from build123d import *

# Parameters (mm, degrees)
F0_R            = 76.2
F1_DEPTH        = 76
F2_R            = 44.704
F3_DEPTH        = 50
F4_R            = 6
F5_DEPTH        = 76
F5_COPIES_COUNT = 6


# Not quite as in the source:
# - a pattern or mirror of a feature is missing from the dataset's text; its kind, count and spacing are read off the source's solid


with BuildPart() as f1:
    # F0 (on Top) → F1 (new body)
    with BuildSketch(Plane.XY):
        Circle(F0_R)
    extrude(amount=F1_DEPTH)

    # F2 (on face) → F3 (cut)
    with BuildSketch(Plane(origin=(0, 0, 0), x_dir=(1, 0, 0), z_dir=(0, 0, -1))):
        Circle(F2_R)
    extrude(amount=-F3_DEPTH, mode=Mode.SUBTRACT)

    # F4 (on face) → F5 (cut)
    with BuildSketch(Plane.XY.offset(76)):
        with Locations((-65, 0)):
            Circle(F4_R)
    f5 = extrude(amount=-F5_DEPTH, mode=Mode.SUBTRACT)

    # F5_copies: F5 ×6 about axis
    f5_copies_axis = Axis((0, 0, 0), (0, 0, 1))
    for i in range(1, F5_COPIES_COUNT):
        add(f5.rotate(f5_copies_axis, i * 360 / F5_COPIES_COUNT), mode=Mode.SUBTRACT)


solid = f1.part
Geometry check sheet. Reference: the model listing, model coordinates, mm. A direction names the side the tool comes from. Coordinates: 2 decimals unless noted, no trailing zeros. Write each loop counter-clockwise with the first axis right and the second up, starting at its lowest first coordinate (ties: lowest second). Pieces come first, ordered by that corner, then holes. Notation, with made-up numbers: (-6, 4) -> (25, 4) arc R21 cw to (25, 22) -> close; hole circle Ø7 at (75, 89.5). An arc over 180 degrees is marked (long way). One line per question, with ' | ' between items.
1. Cross-section at D-D on x = -32.5. Record the cut outline in (y, z).
Answers:
outline: (-68.92, 0) -> (-62.29, 0) -> (-62.29, 76) -> (-68.92, 76) -> close; (-50.29, 0) -> (-30.7, 0) -> (-30.7, 50) -> (30.7, 50) -> (30.7, 0) -> (50.29, 0) -> (50.29, 76) -> (-50.29, 76) -> close; (62.29, 0) -> (68.92, 0) -> (68.92, 76) -> (62.29, 76) -> close
2. Depth check by flat-ended pin: pin 1 Ø8 at (x, z) = (32, 53) entering from -Y; pin 2 Ø2 at (y, z) = (34, 18) entering from +X; pin 3 Ø8 at (x, y) = (38.5, 5) entering from -Z. Enter the tip coordinate at first touch or a pass-through.
Answers:
pin 1: stops at y = -70.87 | pin 2: stops at x = 68.68 | pin 3: stops at z = 50
3. Thickness scan on probe 1 along X at (y, z) = (-0.5, 12); probe 2 along Y at (x, z) = (0, 28); probe 3 along X at (y, z) = (3, 27). Record the ranges inside material, lowest first. Write a range as from..to.
Answers:
probe 1: x = -76.2..-70.98, -59.02..-44.7, 44.7..59.02, 70.98..76.2 | probe 2: y = -76.2..-44.7, 44.7..76.2 | probe 3: x = -76.14..-70.2, -59.8..-44.6, 44.6..59.8, 70.2..76.14
4. Set-up check for faces 4 (the cylindrical face through (-35.476, 27.202, 24.65)), 5 (the cylindrical face through (27.74, 52.64, 38.53)): record each of +Z, -Z, +X, -X, +Y, -Y from which the full face is reachable in a straight line by a thin tool's end or side.
Answers:
face 4: -Z | face 5: +Z, -Z
5. Cross-section at C-C on z = 16.5. Record the cut outline in (x, y).
Answers:
outline: circle Ø152.4 at (0, 0); hole circle Ø12 at (-65, 0); hole circle Ø89.41 at (0, 0); hole circle Ø12 at (-32.5, -56.29); hole circle Ø12 at (-32.5, 56.29); hole circle Ø12 at (32.5, -56.29); hole circle Ø12 at (32.5, 56.29); hole circle Ø12 at (65, 0)
6. Draft check along Y on faces 1 (the cylindrical face through (-60.47, -46.367, 37.468)), 2 (the flat face through (33, -33, 0)), 3 (the flat face through (-1, -1, 50)). Enter one of: +Y half, -Y half, draft (parallel to the pull), parting line (faces both ways), or undercut.
Answers:
face 1: parting line | face 2: draft | face 3: undercut
7. Cross-section at A-A on y = 0. Record the cut outline in (x, z).
Answers:
outline: (-76.2, 0) -> (-71, 0) -> (-71, 76) -> (-76.2, 76) -> close; (-59, 0) -> (-44.7, 0) -> (-44.7, 50) -> (44.7, 50) -> (44.7, 0) -> (59, 0) -> (59, 76) -> (-59, 76) -> close; (71, 0) -> (76.2, 0) -> (76.2, 76) -> (71, 76) -> close
8. Cross-section at B-B on x = 65. Record the cut outline in (y, z), and give its area (3 significant figures).
Answers:
outline: (-39.77, 0) -> (-6, 0) -> (-6, 76) -> (-39.77, 76) -> close; (6, 0) -> (39.77, 0) -> (39.77, 76) -> (6, 76) -> close | area: 5,130 mm²
